Answer from the drawing. Dimensions are ordinates in mm from the lowest x, y and z of the part. A direction names the side the tool comes from. Give positions to 0.01 mm unless a question says otherwise; leave off trailing zeros. Write each loop counter-clockwise with the first axis right and the second up, starting at its lowest first coordinate (ties: lowest second). Pieces come first, ordered by that corner, then holes. Notation, with made-up numbers: M -24.75,77.5 L 7.25,77.5 A33 cw 7.25,115.5 Z; hole C 59,-11 d3. An arc over 180 degrees is marked long. Answer as a JSON object with one key per item and string values.
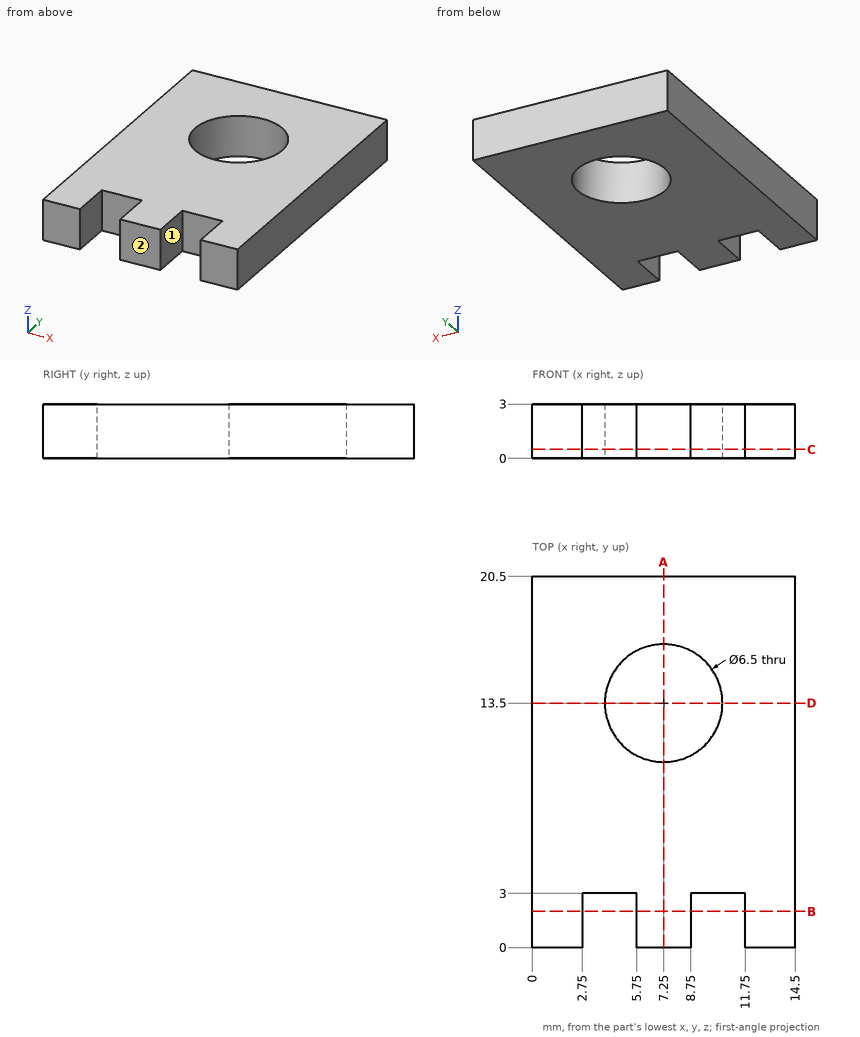
1. A cutting plane is placed at A-A, the plane x = 7.25. Give the vertices of the cut face in (y, z).
Verdict:
{"outline": "M 0,0 L 10.25,0 L 10.25,3 L 0,3 Z; M 16.75,0 L 20.5,0 L 20.5,3 L 16.75,3 Z"}
2. Consider line 1 along Y through (x, z) = (7.25, 1.25); line 2 along Y through (x, z) = (6, 1.55); line 3 along Y through (x, z) = (3, 0.85). Determine where each line is inside the solid, lowest interval first.
Verdict:
{"line 1": "y = 0 to 10.25, 16.75 to 20.5", "line 2": "y = 0 to 10.5, 16.5 to 20.5", "line 3": "y = 3 to 20.5"}
3. Flat-ended cylindrical pins translate along their axes: pin 1 (2 mm diameter, centred on x = 8.5, y = 14.5, fed in from -Z); pin 2 (0.9 mm diameter, centred on x = 10, z = 1.5, fed in from -Y). Find the tip coordinate at first contact, or state that the pin passes through.
Verdict:
{"pin 1": "passes through", "pin 2": "stops at y = 3"}
4. A cutting plane is placed at D-D, the plane y = 13.5. Give the vertices of the cut face in (x, z).
Verdict:
{"outline": "M 0,0 L 4,0 L 4,3 L 0,3 Z; M 10.5,0 L 14.5,0 L 14.5,3 L 10.5,3 Z"}
5. A cutting plane is placed at B-B, the plane y = 2. Give the vertices of the cut face in (x, z).
Verdict:
{"outline": "M 0,0 L 2.75,0 L 2.75,3 L 0,3 Z; M 5.75,0 L 8.75,0 L 8.75,3 L 5.75,3 Z; M 11.75,0 L 14.5,0 L 14.5,3 L 11.75,3 Z"}
6. For the marked faces 1 and 2, determine the directions among +Z, -Z, +X, -X, +Y, -Y from which every point of the face is accessible in a straight line to the end or side of a thin tool.
Verdict:
{"face 1": "+Z, -Z, -Y", "face 2": "+Z, -Z, +X, -X, -Y"}
7. A cutting plane is placed at C-C, the plane z = 0.5. Give the vertices of the cut face in (x, y).
Verdict:
{"outline": "M 0,0 L 2.75,0 L 2.75,3 L 5.75,3 L 5.75,0 L 8.75,0 L 8.75,3 L 11.75,3 L 11.75,0 L 14.5,0 L 14.5,20.5 L 0,20.5 Z; hole C 7.25,13.5 d6.5"}
